Job drawing, mm, ordinate dimensions from the low corner. One solid piece. Round coordinates to 2 decimals unless told otherwise and drop trailing zeros. Order: outer loops, then holes, each group sorted by start corner. A loop starts at its lowest first (then second) coordinate and runs counter-clockwise, first axis right, second up. Notation, with made-up numbers: M 38.25,19 L 93.25,19 A24 cw 93.25,34 Z; hole C -4.75,-21.5 d1. An arc over 180 degrees is marked long. Answer as a JSON object with one key per item and string values. Group by question number.
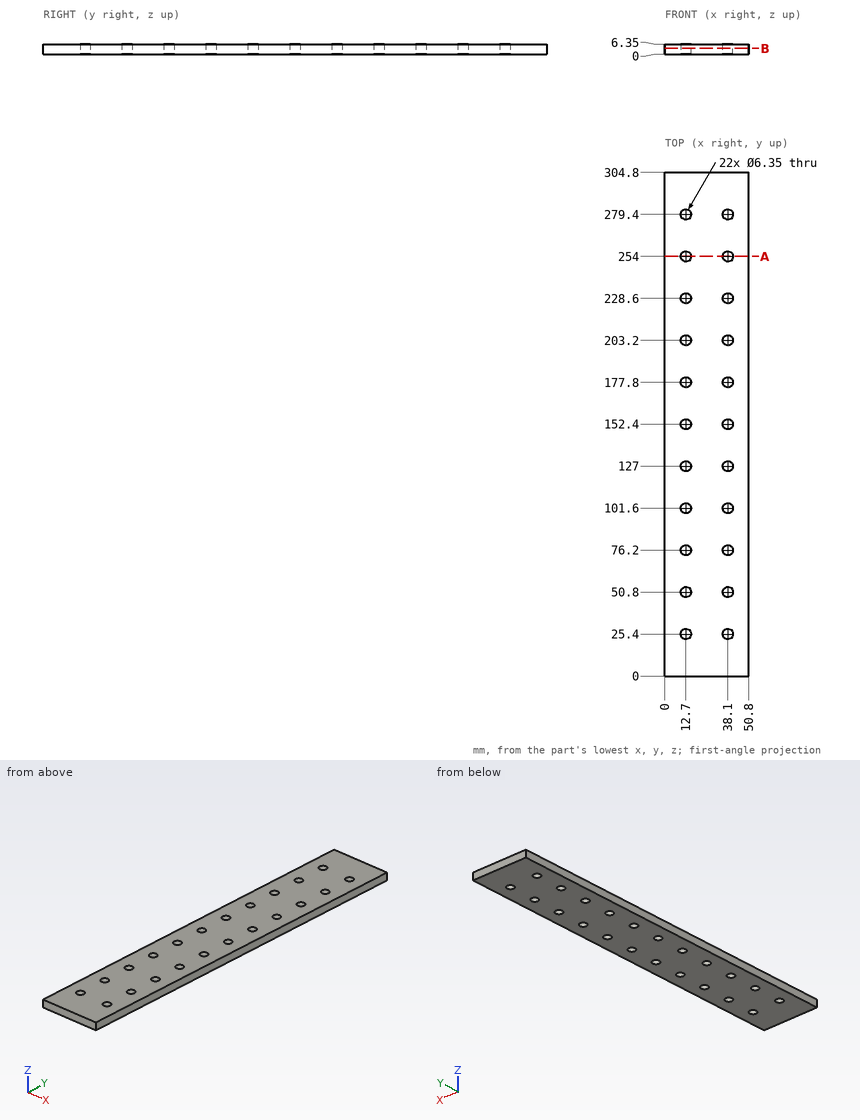
Item 1: Drill centre lines: line 1 (X direction, y = 203.2, z = 4) (3 decimals); line 2 (X direction, y = 228, z = 5.5). Where is each one in solid material? Low to high. Write a range as [from, to].
Item 2: Cut at A-A, the plane y = 254. Give the cut face in (x, z) (3 decimals).
Item 3: Cut at B-B, the plane z = 3.75. Give the number of separate pieces and of enclosed holes in the cut face, and give its area (3 significant figures).
Item 4: Flat gauge pin, fed straight in: pin 1 Ø5 at (x, y) = (38.1, 101.6) entering from -Z. Where does the tip first touch, or does it go through?
Response values:
{
 "1": {"line 1": "[0, 9.525], [15.875, 34.925], [41.275, 50.8]", "line 2": "[0, 9.58], [15.82, 34.98], [41.22, 50.8]"},
 "2": {"outline": "M 0,0 L 9.525,0 L 9.525,6.35 L 0,6.35 Z; M 15.875,0 L 34.925,0 L 34.925,6.35 L 15.875,6.35 Z; M 41.275,0 L 50.8,0 L 50.8,6.35 L 41.275,6.35 Z"},
 "3": {"separate pieces": "1", "enclosed holes": "22", "area": "14,800 mm^2"},
 "4": {"pin 1": "through"}
}
